Part model, mm, in its own coordinate system. A direction names the side the tool comes from. Give positions to 0.01 mm unless a question says otherwise; leave off trailing zeros. Order: outer loops, then holes, each group sorted by start corner. A loop starts at its lowest first (then second) coordinate and runs counter-clockwise, first axis right, second up.
1. Drop flat-ended pins along their axis: pin 1 Ø4 at (x, y) = (-75, 5.5) entering from +Z; pin 2 Ø6 at (y, z) = (5.5, -29) entering from -X; pin 3 Ø1.8 at (y, z) = (7, -6) entering from -X. Give the stop position or say it passes through.
2. Slice it at D-D on z = -21. List the corners of the cut face in (x, y), and give its area (3 significant figures).
3. Slice it at B-B on z = -49. List the corners of the cut face in (x, y), and give its area (3 significant figures).
4. Probe line 1 (X direction, y = 8.75, z = -62); line 2 (X direction, y = 11.5, z = -46.5); line 3 (X direction, y = 11.25, z = -40.5). List the from-to ranges inside material, lowest first.
5. Slice it at A-A on y = 9.25. List the corners of the cut face in (x, z).
6. Mould opens along X. For faces 4 (the flat face through (43, 6, -6)), 5 (the flat face through (102.02, 5.92, -51.8)), 6 (the flat face through (-2, 0, -53)) say: +X half, -X half, draft (parallel to the pull), parting line (faces both ways), or undercut.
7. Slice it at C-C on x = 62.5. List the corners of the cut face in (y, z), and give its area (3 significant figures).
8. Which spindle directions (+Z, -Z, +X, -X, +Y, -Y) get a long thin tool onto all of the face, cutting with end or side? Do faces 1 (the flat face through (57, 6, -12)), 2 (the flat face through (-43, 6, -6)), 3 (the flat face through (70, 6, -34)). Say none if no direction does.
from build123d import *

# Parameters (mm, degrees)
T_LE_DE_BASE_PLI_E1_DEPTH = 12
CONG_1_R                  = 10
CONG_2_R                  = 3


# Sheet-metal steps are written as plain solids
with BuildPart() as part:
    # Esquisse1 → Tôle de base pliée1 (new body)
    with BuildSketch(Plane(origin=(0, 0, 0), x_dir=(1, 0, 0), z_dir=(0, 1, 0))):
        with BuildLine():
            Line((0, 0), (0, 85))
            Line((0, 85), (147.915516427, 85))
            ThreePointArc((147.915516427, 85), (136.110968197, 61.894088575), (120.726964676, 41))
            Line((120.726964676, 41), (70, 70.287226711))
            Line((70, 70.287226711), (70, 12))
            Line((70, 12), (43, 12))
            Line((43, 12), (43, 0))
            Line((43, 0), (0, 0))
        make_face()
    extrude(amount=T_LE_DE_BASE_PLI_E1_DEPTH)

    # Congé1
    cong_1_edges = [part.edges().sort_by_distance(p)[0] for p in [
        (70, 6, -70.287226711),
    ]]
    fillet(cong_1_edges, radius=CONG_1_R)

    # Congé2
    cong_2_edges = [part.edges().sort_by_distance(p)[0] for p in [
        (147.915516427, 6, -85),
        (120.726964676, 6, -41),
        (70, 6, -12),
        (43, 6, -12),
        (43, 6, 0),
    ]]
    fillet(cong_2_edges, radius=CONG_2_R)

    # Symétrie1: part across plane


with BuildPart() as part_1:
    add(part.part)
    add(part.part.mirror(Plane(origin=(0, 12, 0), x_dir=(0, 0, 1), z_dir=(1, 0, 0))))


solid = part_1.part
Data:
1. pin 1: stops at z = -60.11
1. pin 2: stops at x = -70
1. pin 3: stops at x = -43
2. outline: (-70, 0) - (70, 0) - (70, 12) - (-70, 12) - close
2. area: 1,680 mm2
3. outline: (-127.24, 0) - (-106.87, 0) - (-106.87, 12) - (-127.24, 12) - close; (-70, 0) - (70, 0) - (70, 12) - (-70, 12) - close; (106.87, 0) - (127.24, 0) - (127.24, 12) - (106.87, 12) - close
3. area: 2,170 mm2
4. line 1: x = -136.18 to -84.29, -75.71 to 75.71, 84.29 to 136.18
4. line 2: x = -125.3 to -111.2, -70 to 70, 111.2 to 125.3
4. line 3: x = -70 to 70
5. outline: (-146.1, -80.78) arc R3 ccw to (-143.36, -85) - (143.36, -85) arc R3 ccw to (146.1, -80.78) arc R160 ccw to (122.36, -42.91) arc R3 ccw to (118.57, -42.25) - (85, -61.63) arc R10 cw to (70, -52.97) - (70, -15) arc R3 ccw to (67, -12) - (46, -12) arc R3 cw to (43, -9) - (43, -3) arc R3 ccw to (40, 0) - (-40, 0) arc R3 ccw to (-43, -3) - (-43, -9) arc R3 cw to (-46, -12) - (-67, -12) arc R3 ccw to (-70, -15) - (-70, -52.97) arc R10 cw to (-85, -61.63) - (-118.57, -42.25) arc R3 ccw to (-122.36, -42.91) arc R160 ccw to start
6. face 4: +X half
6. face 5: undercut
6. face 6: draft
7. outline: (0, -85) - (12, -85) - (12, -12) - (0, -12) - close
7. area: 876 mm2
8. face 1: +Z, +X, +Y, -Y
8. face 2: +Z, -X, +Y, -Y
8. face 3: +Z, +Y, -Y
